Geometry check sheet. Reference: drawing and pictorial views, mm from the part's lowest x, y, z. A direction names the side the tool comes from. Round coordinates to 2 decimals unless told otherwise and drop trailing zeros. Write each loop counter-clockwise with the first axis right and the second up, starting at its lowest first coordinate (ties: lowest second). Pieces come first, ordered by that corner, then holes. Notation, with made-up numbers: (89.25, 80.25) - (95.25, 80.25) arc R20 ccw to (95.25, 110.25) - close; hole circle Ø5 at (36.25, 70). An arc over 180 degrees is marked (long way). Return JSON: item names as keys, results as strings.
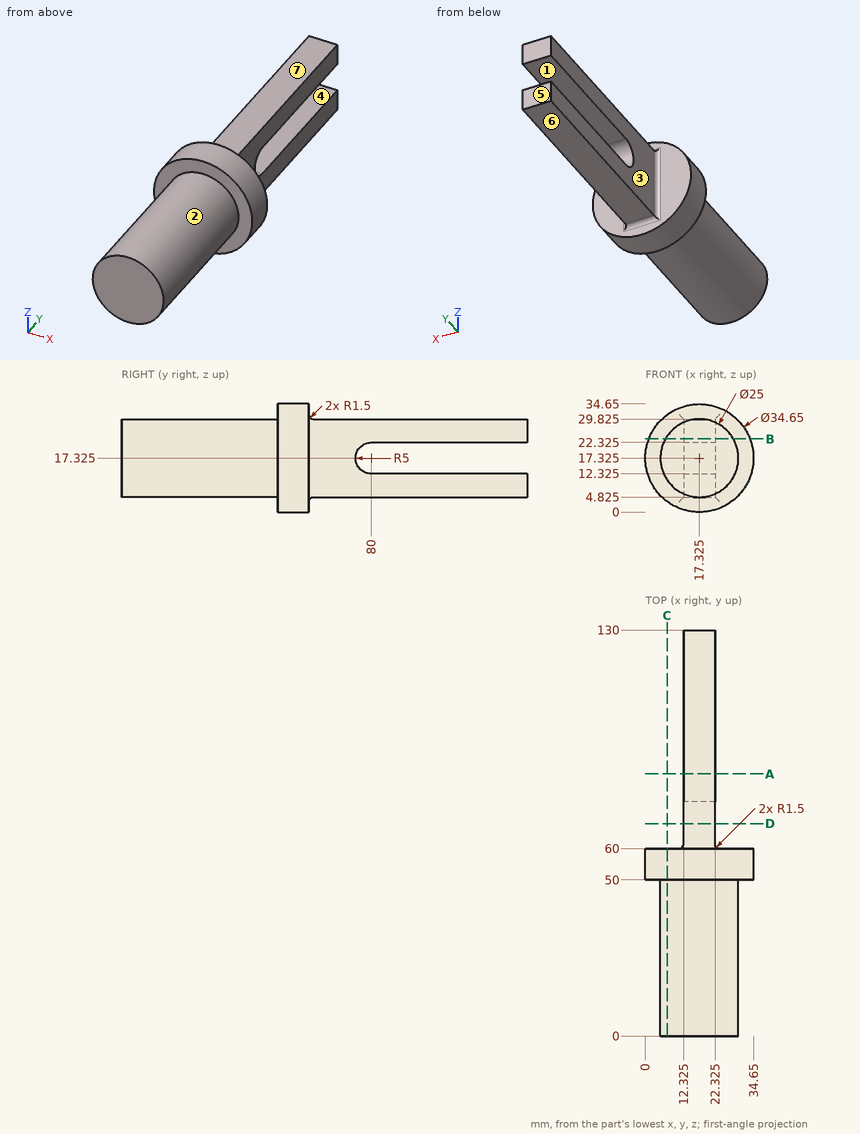
(1) Section check C-C, the plane x = 7. Enter the section's corners in (y, z), plus the area to 3 significant figures.
Response values:
{"outline": "(0, 10.28) - (50, 10.28) - (50, 3.41) - (60, 3.41) - (60, 31.24) - (50, 31.24) - (50, 24.37) - (0, 24.37) - close", "area": "983 mm^2"}
(2) Section check A-A, the plane y = 84. Enter the section's corners in (x, z) (3 decimals).
Response values:
{"outline": "(12.325, 4.825) - (22.325, 4.825) - (22.325, 12.325) - (12.325, 12.325) - close; (12.325, 22.325) - (22.325, 22.325) - (22.325, 29.825) - (12.325, 29.825) - close"}
(3) Section check B-B, the plane z = 23.5. Enter the section's corners in (x, y) (3 decimals).
Response values:
{"outline": "(1.138, 50) - (6.457, 50) - (6.457, 0) - (28.193, 0) - (28.193, 50) - (33.512, 50) - (33.512, 60) - (23.825, 60) arc R1.5 cw to (22.325, 61.5) - (22.325, 130) - (12.325, 130) - (12.325, 61.5) arc R1.5 cw to (10.825, 60) - (1.138, 60) - close"}
(4) Gauge pin test, flat ends, axial feed: pin 1 (11 mm diameter, centred on x = 17, y = 102.5, fed in from +Z) (3 decimals); pin 2 (3 mm diameter, centred on x = 16, z = 19, fed in from +Y); pin 3 (12.5 mm diameter, centred on y = 83, z = 16, fed in from -X) (3 decimals). Record the tip position at first contact, or that the pin passes through.
Response values:
{"pin 1": "stops at z = 29.825", "pin 2": "stops at y = 76.14", "pin 3": "stops at x = 12.325"}
(5) Section check D-D, the plane y = 68. Enter the section's corners in (x, z) (3 decimals), plus the area to 3 significant figures.
Response values:
{"outline": "(12.325, 4.825) - (22.325, 4.825) - (22.325, 29.825) - (12.325, 29.825) - close", "area": "250 mm^2"}
(6) Material ranges on line 1 along Z through (x, y) = (19.5, 113) (3 decimals); line 2 along Y through (x, z) = (26.5, 18.5); line 3 along Y through (x, z) = (6.5, 10), recorded low to high. Write a range as [from, to].
Response values:
{"line 1": "z = [4.825, 12.325], [22.325, 29.825]", "line 2": "y = [0, 60]", "line 3": "y = [50, 60]"}
(7) Release check for a two-part mould opening along Z. For the marked faces 1, 2, 3 and 4 record: pulls with the +Z half, pulls with the -Z half, needs draft (parallel to the pull), parting line crosses it, or undercut.
Response values:
{"face 1": "undercut", "face 2": "parting line crosses it", "face 3": "needs draft", "face 4": "undercut"}
(8) Access from +Z, -Z, +X, -X, +Y, -Y to the whole of each face (thin tool, end or side, straight path). Record for the marked faces 5, 6 and 7.
Response values:
{"face 5": "+Z, -Z, +X, -X, +Y", "face 6": "-Z, +X, -X, +Y", "face 7": "+Z, +X, -X, +Y"}
